Source: CAD feature listing. Evaluate the final solid. Frame: model axes, mm. A direction names the side the tool comes from. Coordinates: 2 decimals unless noted, no trailing zeros. Order: outer loops, then holes, each group sorted by start corner. A loop starts at its lowest first (then second) coordinate and runs counter-clockwise, first axis right, second up. Notation, with made-up numbers: (-15, 24.5) - (12, 24.5) arc R20 cw to (12, 59.5) - close; hole circle Ø10 at (50, 63). An arc over 180 degrees is marked (long way). One line per question, with ' | ' between items. Start each with the question number.
(1) Section D-D (y = -11.5). Return the cut outline in (x, z), then the cut area to 3 significant figures.
(2) Section A-A (z = 24). Return the cut outline in (x, y).
(3) Section C-C (y = -4.5). Return the cut outline in (x, z).
(4) Line query: line 1 along X through (y, z) = (5.25, 20.75); line 2 along Y through (x, z) = (20.5, 21.75); line 3 along Z through (x, y) = (10, -11.5). Output: solid intervals per line, ascending.
(5) Contact query for flat-ended pins moving along their axis: P1, Ø4, axis at y = -2, z = 21, coming from the +X side; P2, Ø2, axis at x = 25, y = -1, coming from the +Z side; P3, Ø5, axis at x = 29, y = -8.5, coming from the +Z side. Output: stop coordinate, or through.
(6) Draft query along Y for faces 3 (the flat face through (20, -15, 12)), 4 (the flat face through (20, 0, 18.75)), 5 (the flat face through (20.28, -10.21, 22.395)). Return one class per face: +Y half, -Y half, draft (parallel to the pull), parting line (faces both ways), or undercut.
(7) Section B-B (x = 28). Return the cut outline in (y, z).
(8) Access query for faces 1 (the flat face through (15, 7.5, 21)), 2 (the flat face through (20, 0, 0)). Directions: +Z, -Z, +X, -X, +Y, -Y. A direction counts if a zero-diameter tool reaches every point of the face in a straight line with its end or side. Return the directions, or none.
from build123d import *

# Parameters (mm, degrees)
F1_DEPTH = 15
F2_DEPTH = 7.5


with BuildPart() as f1:
    # F0 (on Front) → F1 (new body, symmetric)
    with BuildSketch(Plane.XZ):
        Polygon((0, 30), (0, 0), (40, 0), (40, 15), (30, 18.75), (10, 18.75), (10, 26.25), align=None)
        Polygon((30, 18.75), (10, 26.25), (10, 18.75), align=None)
    extrude(amount=F1_DEPTH, both=True)

    # F0 (on Front) → F2 (cut, symmetric)
    with BuildSketch(Plane.XZ):
        Polygon((30, 18.75), (10, 26.25), (10, 18.75), align=None)
    extrude(amount=F2_DEPTH, both=True, mode=Mode.SUBTRACT)


solid = f1.part
Response values:
1) outline: (0, 0) - (40, 0) - (40, 15) - (0, 30) - close | area: 900 mm²
2) outline: (0, -15) - (16, -15) - (16, -7.5) - (10, -7.5) - (10, 7.5) - (16, 7.5) - (16, 15) - (0, 15) - close
3) outline: (0, 0) - (40, 0) - (40, 15) - (30, 18.75) - (10, 18.75) - (10, 26.25) - (0, 30) - close
4) line 1: x = 0 to 10 | line 2: y = -15 to -7.5, 7.5 to 15 | line 3: z = 0 to 26.25
5) P1: stops at x = 10 | P2: stops at z = 18.75 | P3: stops at z = 20.06
6) face 3: -Y half | face 4: undercut | face 5: draft
7) outline: (-15, 0) - (15, 0) - (15, 19.5) - (7.5, 19.5) - (7.5, 18.75) - (-7.5, 18.75) - (-7.5, 19.5) - (-15, 19.5) - close
8) face 1: +Z, +X | face 2: -Z, +X, -X, +Y, -Y
